Verification items for the finished model (mm, model axes). Face numbers are marked on the shaded views. Coordinates: 2 decimals unless noted, no trailing zeros. Order: outer loops, then holes, each group sorted by start corner. A loop starts at its lowest first (then second) coordinate and runs counter-clockwise, first axis right, second up. Notation, with made-up numbers: M 8.25,-26.75 L 20.25,-26.75 A27 ccw 20.25,8.25 Z; hole C 43,73.25 d10. An arc over 180 degrees is marked long. Return JSON: item names as keys, results as strings.
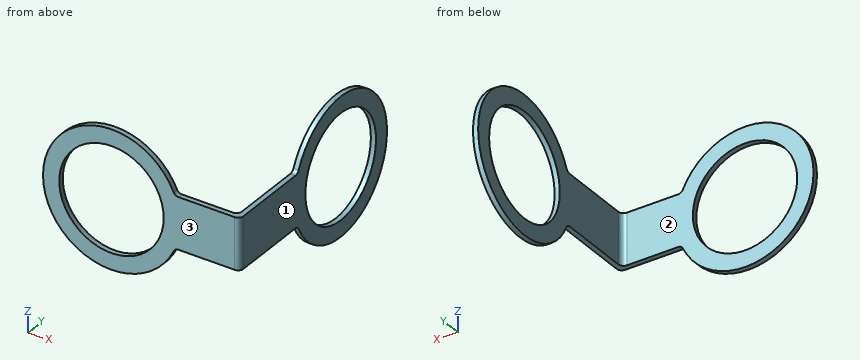
```python
from build123d import *

# Parameters (mm, degrees)
SKETCH1_R           = 40
SKETCH1_R_2         = 30.5
BOSS_EXTRUDE1_DEPTH = 3
SKETCH2_W           = 40
SKETCH2_H           = 30
BOSS_EXTRUDE2_DEPTH = 3
SKETCH3_R           = 30.5
BOSS_EXTRUDE3_DEPTH = 3
FILLET1_R           = 3
FILLET2_R           = 3


with BuildPart() as part:
    # Sketch1 → Boss-Extrude1 (new body)
    with BuildSketch(Plane(origin=(0, 0, 0), x_dir=(1, 0, 0), z_dir=(0, 1, 0))):
        Circle(SKETCH1_R)
        Circle(SKETCH1_R_2, mode=Mode.SUBTRACT)
    extrude(amount=BOSS_EXTRUDE1_DEPTH)

    # Sketch2 → Boss-Extrude2 (add)
    with BuildSketch(Plane(origin=(0, 3, 0), x_dir=(1, 0, 0), z_dir=(0, 1, 0))):
        with Locations((55, 0)):
            Rectangle(SKETCH2_W, SKETCH2_H)
    extrude(amount=-BOSS_EXTRUDE2_DEPTH)

    # Sketch3 → Boss-Extrude3 (add)
    with BuildSketch(Plane(origin=(75, 0, 0), x_dir=(0, 0, -1), z_dir=(1, 0, 0))):
        with BuildLine():
            Line((-15, 0), (15, 0))
            Line((15, 0), (15, 50))
            ThreePointArc((15, 50), (0, 127.080992435), (-15, 50))
            Line((-15, 50), (-15, 0))
        make_face()
        with Locations((0, 87.080992435)):
            Circle(SKETCH3_R, mode=Mode.SUBTRACT)
    extrude(amount=-BOSS_EXTRUDE3_DEPTH)

    # Fillet1
    fillet1_edges = [part.edges().sort_by_distance(p)[0] for p in [
        (37.080992435, 1.5, 15),
        (37.080992435, 1.5, -15),
        (73.5, 50, 15),
        (73.5, 50, -15),
    ]]
    fillet(fillet1_edges, radius=FILLET1_R)

    # Fillet2
    fillet2_edges = [part.edges().sort_by_distance(p)[0] for p in [
        (75, 0, 0),
        (72, 3, 0),
    ]]
    fillet(fillet2_edges, radius=FILLET2_R)


solid = part.part
```
Q1. Cross-section at B-B, the plane z = 0. Record the boundary of the cut face in (x, y).
Values:
{"outline": "M -40,0 L -30.5,0 L -30.5,3 L -40,3 Z; M 30.5,0 L 72,0 A3 ccw 75,3 L 75,56.58 L 72,56.58 L 72,6 A3 cw 69,3 L 30.5,3 Z; M 72,117.58 L 75,117.58 L 75,127.08 L 72,127.08 Z"}
Q2. Cross-section at A-A, the plane x = 0. Record the boundary of the cut face in (y, z).
Values:
{"outline": "M 0,-40 L 3,-40 L 3,-30.5 L 0,-30.5 Z; M 0,30.5 L 3,30.5 L 3,40 L 0,40 Z"}
Q3. Material ranges on line 1 along Y through (x, z) = (-26.5, 19.5); line 2 along X through (y, z) = (64, 30); line 3 along X through (y, z) = (1.95, 0), recorded low to high.
Values:
{"line 1": "0 to 3", "line 2": "72 to 75", "line 3": "-40 to -30.5, 30.5 to 74.81"}
Q4. Go/stop test with flat-tipped pins: pin 1 (8 mm diameter, centred on y = 34.5, z = -0.5, fed in from -X); pin 2 (6 mm diameter, centred on x = 27.5, z = 27, fed in from +Y). Record where each tip stops, or that it passes through.
Values:
{"pin 1": "x = 72", "pin 2": "y = 3"}
Q5. Cross-section at D-D, the plane z = -21.5. Record the boundary of the cut face in (x, y), and give its area (3 significant figures).
Values:
{"outline": "M -33.73,0 L -21.63,0 L -21.63,3 L -33.73,3 Z; M 21.63,0 L 33.73,0 L 33.73,3 L 21.63,3 Z; M 72,53.35 L 75,53.35 L 75,65.45 L 72,65.45 Z; M 72,108.71 L 75,108.71 L 75,120.81 L 72,120.81 Z", "area": "145 mm^2"}
Q6. Cross-section at C-C, the plane y = 106. Record the boundary of the cut face in (x, z), and give its area (3 significant figures).
Values:
{"outline": "M 72,-35.24 L 75,-35.24 L 75,-23.92 L 72,-23.92 Z; M 72,23.92 L 75,23.92 L 75,35.24 L 72,35.24 Z", "area": "67.9 mm^2"}
Q7. Draft check along Y on the marked faces 1, 2 and 3. Enter one of: pulls with the +Y half, pulls with the -Y half, needs draft (parallel to the pull), parting line crosses it, or undercut.
Values:
{"face 1": "needs draft", "face 2": "pulls with the +Y half", "face 3": "pulls with the -Y half"}
